Build history of the part. All positions in model axes, mm. Face numbers are marked on the shaded views. A direction names the side the tool comes from. Give positions to 0.01 mm unless a question says otherwise; leave off trailing zeros. Order: outer loops, then holes, each group sorted by start corner. A loop starts at its lowest first (then second) coordinate and runs counter-clockwise, first axis right, second up. Notation, with made-up numbers: (-31.5, 74) - (-14.5, 74) arc R31 ccw to (-14.5, 100) - close; hole circle Ø10 at (8.25, 70). An arc over 180 degrees is marked (long way). Answer in a Markdown table with one row per item.
```python
from build123d import *

# Parameters (mm, degrees)
BOSS_EXTRUDE1_DEPTH = 47.625
CUT_EXTRUDE1_REACH  = 5.175
SKETCH2_R           = 2.0193


with BuildPart() as part:
    # Sketch1 → Boss-Extrude1 (new body)
    with BuildSketch(Plane(origin=(0, 0, 0), x_dir=(0, 0, -1), z_dir=(1, 0, 0))):
        Polygon((3.175, 3.175), (3.175, 25.4), (0, 25.4), (0, 0), (44.45, 0), (44.45, 3.175), align=None)
    extrude(amount=BOSS_EXTRUDE1_DEPTH)

    # Sketch2 → Cut-Extrude1 (cut, up to next)
    with BuildSketch(Plane(origin=(0, 3.175, 0), x_dir=(1, 0, 0), z_dir=(0, 1, 0)), mode=Mode.PRIVATE) as cut_extrude1_sk1:
        with Locations((11.1125, 23.029)):
            Circle(SKETCH2_R)
    cut_extrude1_tool1 = extrude(cut_extrude1_sk1.sketch, amount=-CUT_EXTRUDE1_REACH, mode=Mode.PRIVATE) & part.part
    add(cut_extrude1_tool1.solids().sort_by_distance((11.1125, 3.175, -23.029))[0], mode=Mode.SUBTRACT)
    # Sketch2 → Cut-Extrude1 (cut, up to next)
    with BuildSketch(Plane(origin=(0, 3.175, 0), x_dir=(1, 0, 0), z_dir=(0, 1, 0)), mode=Mode.PRIVATE) as cut_extrude1_sk2:
        with Locations((11.1125, 35.729)):
            Circle(SKETCH2_R)
    cut_extrude1_tool2 = extrude(cut_extrude1_sk2.sketch, amount=-CUT_EXTRUDE1_REACH, mode=Mode.PRIVATE) & part.part
    add(cut_extrude1_tool2.solids().sort_by_distance((11.1125, 3.175, -35.729))[0], mode=Mode.SUBTRACT)
    # Sketch2 → Cut-Extrude1 (cut, up to next)
    with BuildSketch(Plane(origin=(0, 3.175, 0), x_dir=(1, 0, 0), z_dir=(0, 1, 0)), mode=Mode.PRIVATE) as cut_extrude1_sk3:
        with Locations((36.5125, 23.029)):
            Circle(SKETCH2_R)
    cut_extrude1_tool3 = extrude(cut_extrude1_sk3.sketch, amount=-CUT_EXTRUDE1_REACH, mode=Mode.PRIVATE) & part.part
    add(cut_extrude1_tool3.solids().sort_by_distance((36.5125, 3.175, -23.029))[0], mode=Mode.SUBTRACT)
    # Sketch2 → Cut-Extrude1 (cut, up to next)
    with BuildSketch(Plane(origin=(0, 3.175, 0), x_dir=(1, 0, 0), z_dir=(0, 1, 0)), mode=Mode.PRIVATE) as cut_extrude1_sk4:
        with Locations((36.5125, 35.729)):
            Circle(SKETCH2_R)
    cut_extrude1_tool4 = extrude(cut_extrude1_sk4.sketch, amount=-CUT_EXTRUDE1_REACH, mode=Mode.PRIVATE) & part.part
    add(cut_extrude1_tool4.solids().sort_by_distance((36.5125, 3.175, -35.729))[0], mode=Mode.SUBTRACT)


solid = part.part
```
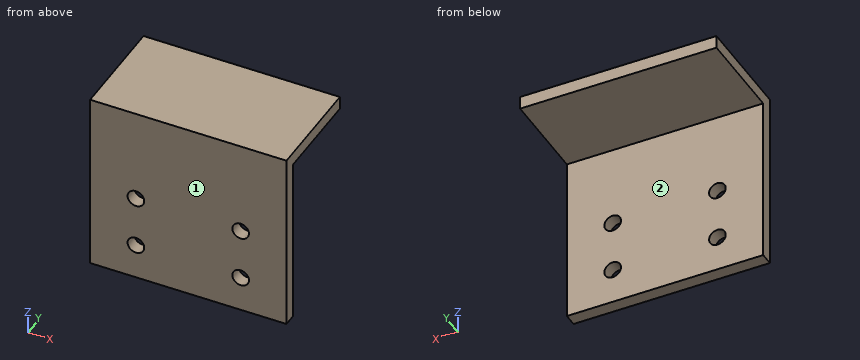
1. Cut at C-C on x = 36. Write the cut outline in (y, z) (3 decimals), and give its area (3 significant figures).
Check result:
| item | result |
|---|---|
| outline | (0, -44.45) - (3.175, -44.45) - (3.175, -37.682) - (0, -37.682) - close; (0, -33.776) - (3.175, -33.776) - (3.175, -24.982) - (0, -24.982) - close; (0, -21.076) - (3.175, -21.076) - (3.175, -3.175) - (25.4, -3.175) - (25.4, 0) - (0, 0) - close |
| area | 187 mm² |
2. Cut at D-D on y = 2. Count the separate pieces of the cut face and the enclosed holes in it, and give its area (3 significant figures).
Check result:
| item | result |
|---|---|
| separate pieces | 1 |
| enclosed holes | 4 |
| area | 2,070 mm² |
3. Cut at B-B on z = -36.5. Write the cut outline in (x, y) (3 decimals), and give its area (3 significant figures).
Check result:
| item | result |
|---|---|
| outline | (0, 0) - (9.246, 0) - (9.246, 3.175) - (0, 3.175) - close; (12.979, 0) - (34.646, 0) - (34.646, 3.175) - (12.979, 3.175) - close; (38.379, 0) - (47.625, 0) - (47.625, 3.175) - (38.379, 3.175) - close |
| area | 128 mm² |
4. Drop flat-ended pins along their axis: P1, Ø3.5, axis at x = 36.51, z = -23.03, coming from the -Y side; P2, Ø12.5, axis at x = 30, z = -29, coming from the +Y side (3 decimals); P3, Ø4, axis at x = 12, y = 15.5, coming from the -Z side (3 decimals). Give the stop position or say it passes through.
Check result:
| item | result |
|---|---|
| P1 | passes through |
| P2 | stops at y = 3.175 |
| P3 | stops at z = -3.175 |
5. Which spindle directions (+Z, -Z, +X, -X, +Y, -Y) get a long thin tool onto all of the face, cutting with end or side? Do the marked faces 1 and 2. Say none if no direction does.
Check result:
| item | result |
|---|---|
| face 1 | +Z, -Z, +X, -X, -Y |
| face 2 | -Z, +X, -X, +Y |
6. Probe line 1 (Y direction, x = 15.5, z = -12) (3 decimals); line 2 (Z direction, x = 36, y = 14) (3 decimals). List the from-to ranges inside material, lowest first.
Check result:
| item | result |
|---|---|
| line 1 | y = 0 to 3.175 |
| line 2 | z = -3.175 to 0 |
7. Cut at A-A on x = 19.5. Write the cut outline in (y, z) (3 decimals), and give its area (3 significant figures).
Check result:
| item | result |
|---|---|
| outline | (0, -44.45) - (3.175, -44.45) - (3.175, -3.175) - (25.4, -3.175) - (25.4, 0) - (0, 0) - close |
| area | 212 mm² |
